CAD build for the part. Positions are in the model's coordinates, mm. Face numbers are marked on the shaded views. A direction names the side the tool comes from. Coordinates: 2 decimals unless noted, no trailing zeros. Loops run counter-clockwise (first coordinate to the right, second up) from the corner with the lowest first, then second, coordinate; pieces in that order, holes last. Notation, with made-up numbers: (38, 52) -> (89, 52) arc R21 cw to (89, 64) -> close; hole circle Ø2 at (62, 67.25). An arc over 180 degrees is marked (long way). Return JSON: item names as keys, results as strings. Group by question number.
(1) Tool access for the marked faces 4 and 5: list every direction of +Z, -Z, +X, -X, +Y, -Y with a clear straight run to the whole face (end or side of a thin tool).
(2) Saw through at C-C on z = 20. Write the cut outline in (x, y), then the cut area to 3 significant figures.
(3) Flat gauge pins, fed straight in: pin 1 Ø4 at (y, z) = (2, 13.5) entering from -X; pin 2 Ø8 at (x, y) = (-3.5, 5.5) entering from +Z; pin 3 Ø4 at (y, z) = (10, 11.5) entering from +X; pin 4 Ø8 at (x, z) = (5.5, 13.5) entering from +Y. Where does each tip first touch, or does it go through?
(4) Saw through at D-D on y = 9. Write the cut outline in (x, z).
(5) Probe L1, parallel to Y at x = -13.5, z = 18.25; L2, parallel to X at y = -1.5, z = 9.5; L3, parallel to X at y = -1.75, z = 16.75. List the from-to ranges inside material, lowest first.
(6) Mould opens along X. For the marked faces 1, 2 and 3 say: pulls with the +X half, pulls with the -X half, needs draft (parallel to the pull), parting line crosses it, or undercut.
(7) Saw through at A-A on x = -1. Write the cut outline in (y, z).
(8) Saw through at B-B on y = 6. Write the cut outline in (x, z), then the cut area to 3 significant figures.
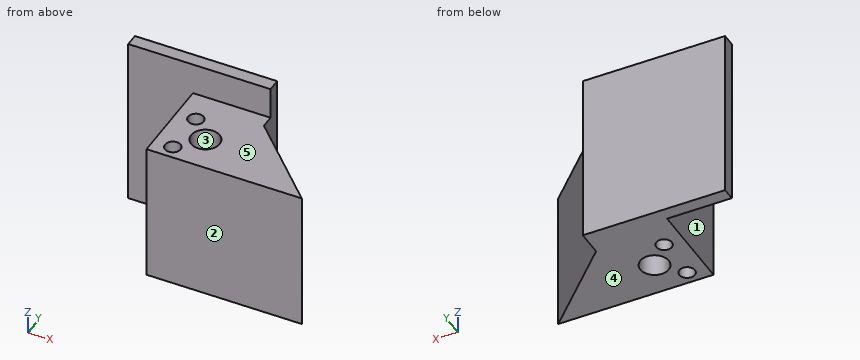
```python
from build123d import *

# Parameters (mm, degrees)
SKETCH_R     = 1.2
SKETCH_R_2   = 2.2
PAD_DEPTH    = 22
SKETCH001_W  = 12
SKETCH001_H  = 22
PAD001_DEPTH = 4
SKETCH002_W  = 2
SKETCH002_H  = 22
PAD002_DEPTH = 10
SKETCH003_W  = 22
SKETCH003_H  = 2
PAD003_DEPTH = 5


with BuildPart() as part:
    # Sketch → Pad (new body)
    with BuildSketch(Plane.XY):
        Polygon((3.852875, 8.478223), (-8.147125, 8.478223), (-8.147125, -3.521777), (15.852875, -3.521777), align=None)
        with Locations((-5.147125, 5.518223)):
            Circle(SKETCH_R, mode=Mode.SUBTRACT)
        with Locations((-5.147125, -1.431777)):
            Circle(SKETCH_R, mode=Mode.SUBTRACT)
        with Locations((-1.907125, 2.078223)):
            Circle(SKETCH_R_2, mode=Mode.SUBTRACT)
    extrude(amount=PAD_DEPTH)

    # Sketch001 (on Face1 of Pad) → Pad001 (join)
    with BuildSketch(Plane(origin=(0, 8.478223, 0), x_dir=(-1, 0, 0), z_dir=(0, 1, 0))):
        with Locations((2.147125, 11)):
            Rectangle(SKETCH001_W, SKETCH001_H)
    extrude(amount=PAD001_DEPTH)

    # Sketch002 (on Face2 of Pad001) → Pad002 (join)
    with BuildSketch(Plane(origin=(-8.147125, 0, 0), x_dir=(0, -1, 0), z_dir=(-1, 0, 0))):
        with Locations((-11.478223, 11)):
            Rectangle(SKETCH002_W, SKETCH002_H)
    extrude(amount=PAD002_DEPTH)

    # Sketch003 (on Face8 of Pad002) → Pad003 (join)
    with BuildSketch(Plane.XY.offset(22)):
        with Locations((-7.147125, 11.478223)):
            Rectangle(SKETCH003_W, SKETCH003_H)
    extrude(amount=PAD003_DEPTH)


solid = part.part
```
Geometry results:
{
 "1": {"face 4": "-Z, +X, -X, +Y, -Y", "face 5": "+Z, +X, -X, -Y"},
 "2": {"outline": "(-18.15, 10.48) -> (-8.15, 10.48) -> (-8.15, -3.52) -> (15.85, -3.52) -> (3.85, 8.48) -> (3.85, 12.48) -> (-18.15, 12.48) -> close; hole circle Ø2.4 at (-5.15, -1.43); hole circle Ø2.4 at (-5.15, 5.52); hole circle Ø4.4 at (-1.91, 2.08)", "area": "260 mm²"},
 "3": {"pin 1": "x = -8.15", "pin 2": "z = 22", "pin 3": "x = 4.33", "pin 4": "y = 12.48"},
 "4": {"outline": "(-8.15, 0) -> (3.85, 0) -> (3.85, 22) -> (-8.15, 22) -> close"},
 "5": {"L1": "10.48 to 12.48", "L2": "-8.15 to -6.35, -3.95 to 13.83", "L3": "-8.15 to -6.3, -3.99 to 14.08"},
 "6": {"face 1": "pulls with the -X half", "face 2": "needs draft", "face 3": "undercut"},
 "7": {"outline": "(-3.52, 0) -> (0.07, 0) -> (0.07, 22) -> (-3.52, 22) -> close; (4.08, 0) -> (12.48, 0) -> (12.48, 27) -> (10.48, 27) -> (10.48, 22) -> (4.08, 22) -> close"},
 "8": {"outline": "(-8.15, 0) -> (-6.25, 0) -> (-6.25, 22) -> (-8.15, 22) -> close; (-4.05, 0) -> (6.33, 0) -> (6.33, 22) -> (-4.05, 22) -> close", "area": "270 mm²"}
}
